The model under review builds one solid part; all positions refer to its coordinate system, in mm. Coordinates: 2 decimals unless noted, no trailing zeros. Loops run counter-clockwise (first coordinate to the right, second up) from the corner with the lowest first, then second, coordinate; pieces in that order, holes last. Notation, with made-up numbers: M 44.25,77 L 76.25,77 A20 cw 76.25,104 Z; hole C -16,43.5 d7. An arc over 180 degrees is marked long. Write item = value, one per line. Start each with the question number.
Q1. We need section B-B on y = 2.05. Count the separate pieces of the cut face and the enclosed holes in it, and give its area (3 significant figures).
Q2. Clearance check with flat-ended pins moving along their axes: pin 1 Ø4 at (x, z) = (55, -65) entering from +Y; pin 2 Ø4.5 at (x, z) = (103.5, -7.5) entering from -Y. State where each tip first meets the part, or that it passes through.
Q3. Wall thickness on probe 1 along X at (y, z) = (1.25, -76); probe 2 along Z at (x, y) = (79.5, 0.7); probe 3 along X at (y, z) = (2.4, -68): over which ranges is each line inside the solid? List them lowest first.
Q4. We need section A-A on x = 72. Give the boundary of the cut face in (y, z).
Q5. We need section D-D on z = -7.5. Give the boundary of the cut face in (x, y), and give its area (3 significant figures).
Q6. We need section C-C on x = 40. Give the boundary of the cut face in (y, z), and give its area (3 significant figures).
from build123d import *

# Parameters (mm, degrees)
SKETCH_1_W          = 110
SKETCH_1_H          = 80
EXTRUDE_1_DEPTH     = 4
SKETCH_2_R          = 2.1
CUT_EXTRUDE_1_DEPTH = 4
FILLET_1_R          = 4
FILLET_2_R          = 5
SKETCH_4_R          = 2.6
CUT_EXTRUDE_2_DEPTH = 10
SKETCH_5_R          = 1.6
CUT_EXTRUDE_3_DEPTH = 10
CUT_EXTRUDE_4_DEPTH = 10
CUT_EXTRUDE_6_REACH = 138.074
SKETCH_8_R          = 2
CUT_EXTRUDE_7_DEPTH = 137.073509545


with BuildPart() as part:
    # 草图1 → 凸台-拉伸1 (new body)
    with BuildSketch(Plane(origin=(0, 0, 0), x_dir=(1, 0, 0), z_dir=(0, 1, 0))):
        with Locations((55, 40)):
            Rectangle(SKETCH_1_W, SKETCH_1_H)
    extrude(amount=EXTRUDE_1_DEPTH)

    # 草图2 → 切除-拉伸1 (cut)
    with BuildSketch(Plane(origin=(0, 4, 0), x_dir=(1, 0, 0), z_dir=(0, 1, 0))):
        with Locations(Location((10, 56.7, 0), (0, 0, 270))):
            Circle(SKETCH_2_R)
        with Locations(Location((40, 56.7, 0), (0, 0, 90))):
            Circle(SKETCH_2_R)
        with Locations(Location((10, 76, 0), (0, 0, 270))):
            Circle(SKETCH_2_R)
        with Locations(Location((40, 76, 0), (0, 0, 90))):
            Circle(SKETCH_2_R)
    extrude(amount=-CUT_EXTRUDE_1_DEPTH, mode=Mode.SUBTRACT)

    # 圆角1
    fillet_1_edges = [part.edges().sort_by_distance(p)[0] for p in [
        (0, 2, -80),
    ]]
    fillet(fillet_1_edges, radius=FILLET_1_R)

    # 圆角2
    fillet_2_edges = [part.edges().sort_by_distance(p)[0] for p in [
        (0, 2, 0),
    ]]
    fillet(fillet_2_edges, radius=FILLET_2_R)

    # 草图4 → 切除-拉伸2 (cut)
    with BuildSketch(Plane(origin=(0, 4, 0), x_dir=(1, 0, 0), z_dir=(0, 1, 0))):
        with Locations(Location((103.5, 47.5, 0), (0, 0, 270))):
            Circle(SKETCH_4_R)
        with Locations(Location((103.5, 72.5, 0), (0, 0, 270))):
            Circle(SKETCH_4_R)
        with Locations(Location((103.5, 7.5, 0), (0, 0, 90))):
            Circle(SKETCH_4_R)
        with Locations(Location((103.5, 32.5, 0), (0, 0, 90))):
            Circle(SKETCH_4_R)
    extrude(amount=-CUT_EXTRUDE_2_DEPTH, mode=Mode.SUBTRACT)

    # 草图5 → 切除-拉伸3 (cut)
    with BuildSketch(Plane.XZ):
        with Locations(Location((55, -65, 0), (0, 0, 270))):
            Circle(SKETCH_5_R)
        with Locations(Location((65, -65, 0), (0, 0, 270))):
            Circle(SKETCH_5_R)
    cut_extrude_3 = extrude(amount=-CUT_EXTRUDE_3_DEPTH, mode=Mode.SUBTRACT)

    # 草图6 → 切除-拉伸4 (cut)
    with BuildSketch(Plane.XZ):
        Polygon((0, -40.5), (75, 0), (0, 0), align=None)
    extrude(amount=-CUT_EXTRUDE_4_DEPTH, mode=Mode.SUBTRACT)

    # 草图8 → 切除-拉伸6 (cut, up to next)
    with BuildSketch(Plane.XZ, mode=Mode.PRIVATE) as cut_extrude_6_sk1:
        with Locations(Location((10, -68, 0), (0, 0, 270))):
            Circle(SKETCH_8_R)
    cut_extrude_6_tool1 = extrude(cut_extrude_6_sk1.sketch, amount=-CUT_EXTRUDE_6_REACH, mode=Mode.PRIVATE) & part.part
    # 草图8 → 切除-拉伸6 (cut, up to next)
    with BuildSketch(Plane.XZ, mode=Mode.PRIVATE) as cut_extrude_6_sk2:
        with Locations(Location((40, -68, 0), (0, 0, 270))):
            Circle(SKETCH_8_R)
    cut_extrude_6_tool2 = extrude(cut_extrude_6_sk2.sketch, amount=-CUT_EXTRUDE_6_REACH, mode=Mode.PRIVATE) & part.part
    add(cut_extrude_6_tool1.solids().sort_by_distance((10, 0, -68))[0], mode=Mode.SUBTRACT)
    add(cut_extrude_6_tool2.solids().sort_by_distance((40, 0, -68))[0], mode=Mode.SUBTRACT)

    # 镜向1: 切除-拉伸3 across plane
    add(cut_extrude_3.mirror(Plane(origin=(0, 0, -45), x_dir=(1, 0, 0), z_dir=(0, 0, -1))), mode=Mode.SUBTRACT)

    # 草图9 → 切除-拉伸7 (cut, through all)
    with BuildSketch(Plane.XZ):
        with BuildLine():
            Line((85, -36.949085991), (50, -36.949085991))
            ThreePointArc((50, -36.949085991), (47.5, -39.449085991), (50, -41.949085991))
            Line((50, -41.949085991), (85, -41.949085991))
            ThreePointArc((85, -41.949085991), (87.5, -39.449085991), (85, -36.949085991))
        make_face()
        with BuildLine():
            Line((85, -51.949085991), (50, -51.949085991))
            ThreePointArc((50, -51.949085991), (47.5, -54.449085991), (50, -56.949085991))
            Line((50, -56.949085991), (85, -56.949085991))
            ThreePointArc((85, -56.949085991), (87.5, -54.449085991), (85, -51.949085991))
        make_face()
    extrude(amount=-CUT_EXTRUDE_7_DEPTH, mode=Mode.SUBTRACT)


solid = part.part
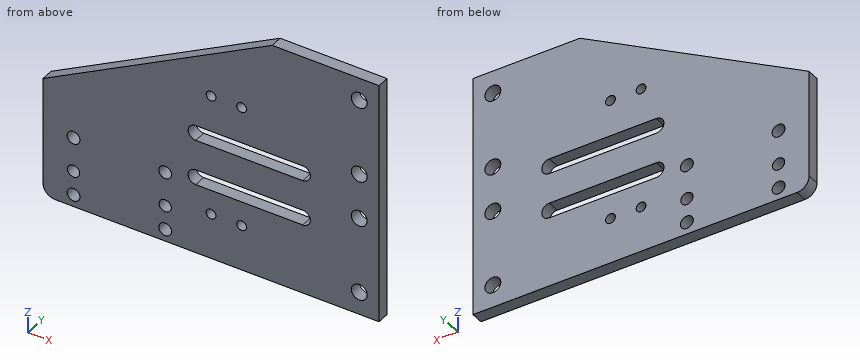
Returned:
q1.separate_pieces = 1
q1.enclosed_holes = 16
q1.area = 6,690 mm^2
q2.pin_1 = 4
q2.pin_2 = through
q3.probe_1 = 0 to 7.9, 12.1 to 37.9, 42.1 to 110
q3.probe_2 = -80 to -56.95, -51.95 to -41.95, -36.95 to 0
q3.probe_3 = 0 to 8, 12 to 38, 42 to 110
q4.outline = M 0,-80 L 4,-80 L 4,-56.95 L 0,-56.95 Z; M 0,-51.95 L 4,-51.95 L 4,-41.95 L 0,-41.95 Z; M 0,-36.95 L 4,-36.95 L 4,-1.62 L 0,-1.62 Z
q5.outline = M 61.11,0 L 100.9,0 L 100.9,4 L 61.11,4 Z; M 106.1,0 L 110,0 L 110,4 L 106.1,4 Z
q5.area = 175 mm^2
q6.outline = M 0,-80 L 4,-80 L 4,-78.1 L 0,-78.1 Z; M 0,-73.9 L 4,-73.9 L 4,-70 L 0,-70 Z; M 0,-66 L 4,-66 L 4,-58.8 L 0,-58.8 Z; M 0,-54.6 L 4,-54.6 L 4,-18.9 L 0,-18.9 Z
q6.area = 195 mm^2
